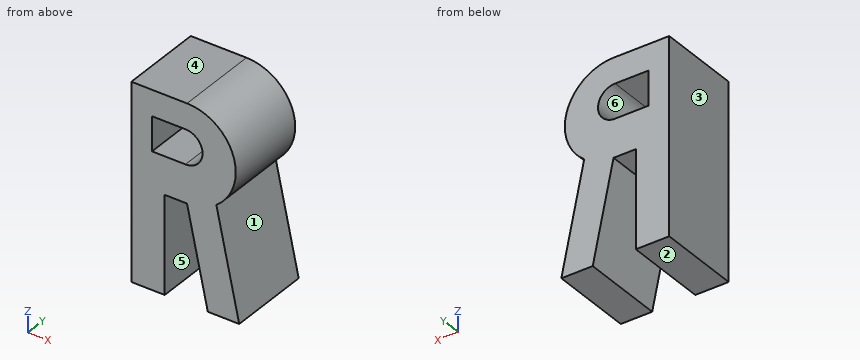
```python
from build123d import *

# Parameters (mm, degrees)
F0_W     = 3.048
F0_H     = 8.89
F1_DEPTH = 7.62
F2_DEPTH = 7.62
F3_W     = 3.048
F3_H     = 3.1197171271
F4_DEPTH = 25.4


# Not quite as in the source:
# - a feature names something its author has since deleted; it is built from what else it names


with BuildPart() as f1:
    # F0 (on Front) → F1 (new body)
    with BuildSketch(Plane.XZ):
        Polygon((-6.9585410112, 8.89), (-12.0385410112, 8.89), (-12.0385410112, 0), (-8.9905410112, 0), (-6.9585410112, 0), align=None)
        with BuildLine():
            ThreePointArc((-4.2838060673, 0.8948143739), (-2.7431762518, 5.8552215946), (-6.9585410112, 8.89))
            Line((-6.9585410112, 8.89), (-6.9585410112, 0))
            ThreePointArc((-6.9585410112, 0), (-5.5483194165, 0.2296352407), (-4.2838060673, 0.8948143739))
        make_face()
        with Locations((-10.5145410112, -4.445)):
            Rectangle(F0_W, F0_H)
    extrude(amount=F1_DEPTH)

    # F0 (on Front) → F2 (join)
    with BuildSketch(Plane.XZ):
        Polygon((-6.9585410112, 8.89), (-12.0385410112, 8.89), (-12.0385410112, 0), (-8.9905410112, 0), (-6.9585410112, 0), align=None)
        with BuildLine():
            ThreePointArc((-4.2838060673, 0.8948143739), (-2.7431762518, 5.8552215946), (-6.9585410112, 8.89))
            Line((-6.9585410112, 8.89), (-6.9585410112, 0))
            ThreePointArc((-6.9585410112, 0), (-5.5483194165, 0.2296352407), (-4.2838060673, 0.8948143739))
        make_face()
        with Locations((-10.5145410112, -4.445)):
            Rectangle(F0_W, F0_H)
        with BuildLine():
            ThreePointArc((-4.2838060673, 0.8948143739), (-5.5483194165, 0.2296352407), (-6.9585410112, 0))
            Line((-6.9585410112, 0), (-5.0608660094, -8.89))
            Line((-5.0608660094, -8.89), (-2.1951224189, -8.89))
            Line((-2.1951224189, -8.89), (-4.2838060673, 0.8948143739))
        make_face()
    extrude(amount=F2_DEPTH)

    # F3 (on face) → F4 (cut)
    with BuildSketch(Plane.XZ.offset(7.62)):
        with Locations((-8.624184413, 4.9824524904)):
            Rectangle(F3_W, F3_H)
        with BuildLine():
            ThreePointArc((-7.100184413, 3.4225939268), (-5.5403258494, 4.9824524904), (-7.100184413, 6.5423110539))
            Line((-7.100184413, 6.5423110539), (-7.100184413, 3.4225939268))
        make_face()
    extrude(amount=-F4_DEPTH, mode=Mode.SUBTRACT)


solid = f1.part
```
Can you work these out from the model? Positions are in its coordinate system, mm. Face numbers are marked on the shaded views. A direction names the side the tool comes from. Give positions to 0.01 mm unless a question says otherwise; leave off trailing zeros. Loops run counter-clockwise (first coordinate to the right, second up) from the corner with the lowest first, then second, coordinate; pieces in that order, holes last. Notation, with made-up numbers: M 27.25,83.5 L 44.25,83.5 A18 ccw 44.25,106.5 Z; hole C -20,-18 d6. An arc over 180 degrees is marked long. One line per question, with ' | ' between items. Start each with the question number.
Q1. For the marked faces 4, 5 and 6, which set-ups out of +Z, -Z, +X, -X, +Y, -Y let a thin tool reach every point of the face, with its end or its side?
Q2. If we section it at C-C (y = -3.75): Please give me the cut outline in (x, z) (3 decimals), plus the area to 3 significant figures.
Q3. If we mould it in two halves opening along Z, with no side actions, what happens to the marked faces 1, 2 and 3? For each: +Z half, -Z half, draft (parallel to the pull), parting line (faces both ways), or undercut.
Q4. If we section it at B-B (z = -6.5): Please give me the cut outline in (x, y), plus the area to 3 significant figures.
Q5. For pin 1 Ø0.6 at (x, y) = (-7.5, -2) entering from -Z; pin 2 Ø4 at (x, z) = (-5, 7) entering from +Y; pin 3 Ø3 at (x, y) = (-5, -1) entering from +Z; pin 4 Ø1.6 at (y, z) = (-2, 5.5) entering from +X, each with a flat end and sliding along its axis, tell me the tip position at first contact or that it passes through.
Q6. If I drill on line 1 (Z direction, x = -8, y = -2.75); line 2 (Z direction, x = -9.5, y = -4.5); line 3 (X direction, y = -3.5, z = -0.25), over which ranges is the centre line in solid material (lowest first)? Write a range as from..to.
Q7. If we section it at A-A (x = -7.5): Please give me the cut outline in (y, z), plus the area to 3 significant figures.
Q8. If we section it at D-D (z = 2.5): Please give me the cut outline in (x, y), plus the area to 3 significant figures.
Computed:
1) face 4: +Z, +X, -X, +Y, -Y | face 5: -Z, +Y, -Y | face 6: +Y, -Y
2) outline: M -12.039,-8.89 L -8.991,-8.89 L -8.991,0 L -6.959,0 L -5.061,-8.89 L -2.195,-8.89 L -4.284,0.895 A4.445 ccw -6.959,8.89 L -12.039,8.89 Z; hole M -10.148,3.423 L -7.1,3.423 A1.56 ccw -7.1,6.542 L -10.148,6.542 Z | area: 116 mm²
3) face 1: undercut | face 2: -Z half | face 3: draft
4) outline: M -12.04,-7.62 L -8.99,-7.62 L -8.99,0 L -12.04,0 Z; M -5.57,-7.62 L -2.71,-7.62 L -2.71,0 L -5.57,0 Z | area: 45.1 mm²
5) pin 1: stops at z = 0 | pin 2: stops at y = 0 | pin 3: stops at z = 8.87 | pin 4: stops at x = -2.52
6) line 1: z = 0..3.42, 6.54..8.89 | line 2: z = -8.89..3.42, 6.54..8.89 | line 3: x = -12.04..-8.99, -6.91..-4.04
7) outline: M -7.62,0 L 0,0 L 0,3.42 L -7.62,3.42 Z; M -7.62,6.54 L 0,6.54 L 0,8.89 L -7.62,8.89 Z | area: 44.0 mm²
8) outline: M -12.04,-7.62 L -2.96,-7.62 L -2.96,0 L -12.04,0 Z | area: 69.2 mm²
